```python
from build123d import *

# Parameters (mm, degrees)
F1_DEPTH     = 2.54
F3_DEPTH     = 2.54
F4_R         = 2.9314454593
F5_R         = 2.8319389427
F6_DEPTH     = 8.89
F8_DEPTH     = 25.4
F9_T1_DEPTH  = 38.1
F9_T3_DEPTH  = 38.1
F9_T5_DEPTH  = 21.5282681004
F9_T7_DEPTH  = 32.0580135728
F9_T9_DEPTH  = 55.7565362009
F9_T11_DEPTH = 34.6970452561
F9_T13_DEPTH = 34.6970452561
F9_T16_ANGLE = 223.4050528115
F9_T21_DEPTH = 49.0985226281
F9_T25_DEPTH = 32.5267907285
F9_T32_DEPTH = 32.0580135728
F9_T37_DEPTH = 49.0985226281
F9_T44_DEPTH = 49.0985226281
F9_T48_DEPTH = 32.0580135728
F9_T56_DEPTH = 32.5267907285
F9_T60_DEPTH = 49.0985226281
F10_R        = 1.4567648878
F10_R_2      = 1.5876943873
F11_DEPTH    = 0.508
F12_R        = 0.6244535606
F12_R_2      = 0.645662674
F13_DEPTH    = 0.254


# Not quite as in the source:
# - a fillet or chamfer that OpenCascade refuses, or shapes differently, is made with other operations: its cross-section is extruded or revolved along the edge and cut away or added


with BuildPart() as f1:
    # F0 (on Front) → F1 (new body)
    with BuildSketch(Plane.XZ):
        Polygon((27.5468391635, 41.7749450469), (-86.7531608365, 41.7749450469), (-86.7531608365, 8.0154541022), (-74.0531608365, 8.0154541022), (-74.0531608365, 29.0749450469), (-35.9531608365, 29.0749450469), (-35.9531608365, 8.0154541022), (-23.2531608365, 8.0154541022), (-23.2531608365, 29.0749450469), (14.8468391635, 29.0749450469), (14.8468391635, 8.0154541022), (27.5468391635, 8.0154541022), align=None)
    extrude(amount=F1_DEPTH)

    # F2 (on face) → F3 (join)
    with BuildSketch(Plane.XY.offset(41.7749450469)):
        with BuildLine():
            Line((27.5468391635, -2.54), (13.0688391635, -2.54))
            ThreePointArc((13.0688391635, -2.54), (20.3078391635, -9.779), (27.5468391635, -2.54))
        make_face()
        with BuildLine():
            Line((-72.2751608365, -2.54), (-86.7531608365, -2.54))
            ThreePointArc((-86.7531608365, -2.54), (-79.5141608365, -9.779), (-72.2751608365, -2.54))
        make_face()
    extrude(amount=-F3_DEPTH)

    # F4 (on face) + F5 (on face) → F6 (join)
    with BuildSketch(Plane(origin=(0, 0, 39.2349450469), x_dir=(1, 0, 0), z_dir=(0, 0, -1))):
        with Locations((-79.5141608365, 6.3278437592)):
            Circle(F4_R)
    with BuildSketch(Plane(origin=(0, 0, 39.2349450469), x_dir=(1, 0, 0), z_dir=(0, 0, -1))):
        with Locations((20.3078391635, 6.6598863341)):
            Circle(F5_R)
    extrude(amount=F6_DEPTH)

    # F7 (on face) → F8 (cut)
    with BuildSketch(Plane.XZ.offset(2.54)):
        with BuildLine():
            Line((-23.2531608365, 8.0154541022), (-23.2531608365, 18.5451995745))
            ThreePointArc((-23.2531608365, 18.5451995745), (-29.6031608365, 21.0747577819), (-35.9531608365, 18.5451995745))
            Line((-35.9531608365, 18.5451995745), (-35.9531608365, 8.0154541022))
            Line((-35.9531608365, 8.0154541022), (-23.2531608365, 8.0154541022))
        make_face()
    extrude(amount=-F8_DEPTH, mode=Mode.SUBTRACT)

    # F9: fillet of radius 5.08 on 11 edges, made by hand

    # F9_s2 → F9_t1 (cut)
    with BuildSketch(Plane.YZ.offset(-23.2531608365)):
        with BuildLine():
            ThreePointArc((0, 33.4743540981), (-0.6805909488, 30.9343540981), (-2.54, 29.0749450469))
            Line((-2.54, 29.0749450469), (0, 29.0749450469))
            Line((0, 29.0749450469), (0, 33.4743540981))
        make_face()
    extrude(amount=F9_T1_DEPTH, mode=Mode.SUBTRACT)

    # F9_s4 → F9_t3 (cut)
    with BuildSketch(Plane.YZ.offset(-74.0531608365)):
        with BuildLine():
            ThreePointArc((0, 33.4743540981), (-0.6805909488, 30.9343540981), (-2.54, 29.0749450469))
            Line((-2.54, 29.0749450469), (0, 29.0749450469))
            Line((0, 29.0749450469), (0, 33.4743540981))
        make_face()
    extrude(amount=F9_T3_DEPTH, mode=Mode.SUBTRACT)

    # F9_s6 → F9_t5 (cut)
    with BuildSketch(Plane.XY.offset(7.5466769465)):
        with BuildLine():
            ThreePointArc((-31.5537517853, 0), (-34.0937517853, -0.6805909488), (-35.9531608365, -2.54))
            Line((-35.9531608365, -2.54), (-35.9531608365, 0))
            Line((-35.9531608365, 0), (-31.5537517853, 0))
        make_face()
        with BuildLine():
            ThreePointArc((-27.6525698878, 0), (-25.1125698878, -0.6805909488), (-23.2531608365, -2.54))
            Line((-23.2531608365, -2.54), (-23.2531608365, 0))
            Line((-23.2531608365, 0), (-27.6525698878, 0))
        make_face()
    extrude(amount=F9_T5_DEPTH, mode=Mode.SUBTRACT)

    # F9_s8 → F9_t7 (cut)
    with BuildSketch(Plane.XY.offset(-2.9830685259)):
        with BuildLine():
            ThreePointArc((19.2462482147, 0), (16.7062482147, -0.6805909488), (14.8468391635, -2.54))
            Line((14.8468391635, -2.54), (14.8468391635, 0))
            Line((14.8468391635, 0), (19.2462482147, 0))
        make_face()
        with BuildLine():
            ThreePointArc((-78.4525698878, 0), (-75.9125698878, -0.6805909488), (-74.0531608365, -2.54))
            Line((-74.0531608365, -2.54), (-74.0531608365, 0))
            Line((-74.0531608365, 0), (-78.4525698878, 0))
        make_face()
    extrude(amount=F9_T7_DEPTH, mode=Mode.SUBTRACT)

    # F9_s10 → F9_t9 (cut)
    with BuildSketch(Plane.XY.offset(-2.9830685259)):
        with BuildLine():
            ThreePointArc((27.5468391635, -2.54), (25.6874301122, -0.6805909488), (23.1474301122, 0))
            Line((23.1474301122, 0), (27.5468391635, 0))
            Line((27.5468391635, 0), (27.5468391635, -2.54))
        make_face()
        with BuildLine():
            ThreePointArc((-86.7531608365, -2.54), (-84.8937517853, -0.6805909488), (-82.3537517853, 0))
            Line((-82.3537517853, 0), (-86.7531608365, 0))
            Line((-86.7531608365, 0), (-86.7531608365, -2.54))
        make_face()
    extrude(amount=F9_T9_DEPTH, mode=Mode.SUBTRACT)

    # F9_s12 → F9_t11 (cut)
    with BuildSketch(Plane.YZ.offset(-97.7516834646)):
        with BuildLine():
            ThreePointArc((0, 12.4148631534), (-0.6805909488, 9.8748631534), (-2.54, 8.0154541022))
            Line((-2.54, 8.0154541022), (0, 8.0154541022))
            Line((0, 8.0154541022), (0, 12.4148631534))
        make_face()
    extrude(amount=F9_T11_DEPTH, mode=Mode.SUBTRACT)

    # F9_s14 → F9_t13 (cut)
    with BuildSketch(Plane.YZ.offset(3.8483165354)):
        with BuildLine():
            ThreePointArc((0, 12.4148631534), (-0.6805909488, 9.8748631534), (-2.54, 8.0154541022))
            Line((-2.54, 8.0154541022), (0, 8.0154541022))
            Line((0, 8.0154541022), (0, 12.4148631534))
        make_face()
    extrude(amount=F9_T13_DEPTH, mode=Mode.SUBTRACT)

    # F9_s15 → F9_t16 (revolve, cut)
    with BuildSketch(Plane(origin=(0.0198149882, 0, 0.0497864763), x_dir=(0, 1, 0), z_dir=(-0.3697877262, 0, -0.929116267))):
        with BuildLine():
            ThreePointArc((0, -18.2485055237), (-0.6805909488, -20.7885055237), (-2.54, -22.6479145749))
            Line((-2.54, -22.6479145749), (0, -22.6479145749))
            Line((0, -22.6479145749), (0, -18.2485055237))
        make_face()
    revolve(axis=Axis((-29.6031608365, 0, 11.8397133801), (0, -1, 0)), revolution_arc=F9_T16_ANGLE, mode=Mode.SUBTRACT)


with BuildPart() as f9_tool19:
    # F9_s20 → F9_t21 (new body)
    with BuildSketch(Plane.YZ.offset(-34.2516834646)):
        with BuildLine():
            ThreePointArc((0, 33.4743540981), (-0.6805909488, 30.9343540981), (-2.54, 29.0749450469))
            Line((-2.54, 29.0749450469), (0, 29.0749450469))
            Line((0, 29.0749450469), (0, 33.4743540981))
        make_face()
    extrude(amount=F9_T21_DEPTH)

    split(bisect_by=Plane.YZ.offset(-23.2531608365), keep=Keep.BOTTOM)


with BuildPart() as f9_tool23:
    # F9_s24 → F9_t25 (new body)
    with BuildSketch(Plane.XY.offset(7.5466769465)):
        with BuildLine():
            ThreePointArc((-27.6525698878, 0), (-25.1125698878, -0.6805909488), (-23.2531608365, -2.54))
            Line((-23.2531608365, -2.54), (-23.2531608365, 0))
            Line((-23.2531608365, 0), (-27.6525698878, 0))
        make_face()
    extrude(amount=F9_T25_DEPTH)

    split(bisect_by=Plane.XY.offset(29.0749450469), keep=Keep.TOP)


with BuildPart() as f9_tool19_1:
    add(f9_tool19.part)

    # F9_t27: intersect F9_tool23
    add(f9_tool23.part, mode=Mode.INTERSECT)


with BuildPart() as f1_1:
    add(f1.part)

    # F9_t17: cut F9_tool19
    add(f9_tool19_1.part, mode=Mode.SUBTRACT)


with BuildPart() as f9_tool30:
    # F9_s31 → F9_t32 (new body)
    with BuildSketch(Plane.XY.offset(40.073467675)):
        with BuildLine():
            ThreePointArc((19.2462482147, 0), (16.7062482147, -0.6805909488), (14.8468391635, -2.54))
            Line((14.8468391635, -2.54), (14.8468391635, 0))
            Line((14.8468391635, 0), (19.2462482147, 0))
        make_face()
    extrude(amount=-F9_T32_DEPTH)

    split(bisect_by=Plane.XY.offset(39.2349450469), keep=Keep.BOTTOM)

    split(bisect_by=Plane.XY.offset(29.0749450469), keep=Keep.TOP)


with BuildPart() as f9_tool35:
    # F9_s36 → F9_t37 (new body)
    with BuildSketch(Plane.YZ.offset(-23.2531608365)):
        with BuildLine():
            ThreePointArc((0, 33.4743540981), (-0.6805909488, 30.9343540981), (-2.54, 29.0749450469))
            Line((-2.54, 29.0749450469), (0, 29.0749450469))
            Line((0, 29.0749450469), (0, 33.4743540981))
        make_face()
    extrude(amount=F9_T37_DEPTH)

    split(bisect_by=Plane.YZ.offset(14.8468391635), keep=Keep.TOP)


with BuildPart() as f9_tool30_1:
    add(f9_tool30.part)

    # F9_t39: intersect F9_tool35
    add(f9_tool35.part, mode=Mode.INTERSECT)


with BuildPart() as f1_2:
    add(f1_1.part)

    # F9_t28: cut F9_tool30
    add(f9_tool30_1.part, mode=Mode.SUBTRACT)


with BuildPart() as f9_tool42:
    # F9_s43 → F9_t44 (new body)
    with BuildSketch(Plane.YZ.offset(-85.0516834646)):
        with BuildLine():
            ThreePointArc((0, 33.4743540981), (-0.6805909488, 30.9343540981), (-2.54, 29.0749450469))
            Line((-2.54, 29.0749450469), (0, 29.0749450469))
            Line((0, 29.0749450469), (0, 33.4743540981))
        make_face()
    extrude(amount=F9_T44_DEPTH)

    split(bisect_by=Plane.YZ.offset(-74.0531608365), keep=Keep.BOTTOM)


with BuildPart() as f9_tool46:
    # F9_s47 → F9_t48 (new body)
    with BuildSketch(Plane.XY.offset(8.0154541022)):
        with BuildLine():
            ThreePointArc((-78.4525698878, 0), (-75.9125698878, -0.6805909488), (-74.0531608365, -2.54))
            Line((-74.0531608365, -2.54), (-74.0531608365, 0))
            Line((-74.0531608365, 0), (-78.4525698878, 0))
        make_face()
    extrude(amount=F9_T48_DEPTH)

    split(bisect_by=Plane.XY.offset(29.0749450469), keep=Keep.TOP)

    split(bisect_by=Plane.XY.offset(39.2349450469), keep=Keep.BOTTOM)


with BuildPart() as f9_tool42_1:
    add(f9_tool42.part)

    # F9_t51: intersect F9_tool46
    add(f9_tool46.part, mode=Mode.INTERSECT)


with BuildPart() as f1_3:
    add(f1_2.part)

    # F9_t40: cut F9_tool42
    add(f9_tool42_1.part, mode=Mode.SUBTRACT)


with BuildPart() as f9_tool54:
    # F9_s55 → F9_t56 (new body)
    with BuildSketch(Plane.XY.offset(40.073467675)):
        with BuildLine():
            ThreePointArc((-31.5537517853, 0), (-34.0937517853, -0.6805909488), (-35.9531608365, -2.54))
            Line((-35.9531608365, -2.54), (-35.9531608365, 0))
            Line((-35.9531608365, 0), (-31.5537517853, 0))
        make_face()
    extrude(amount=-F9_T56_DEPTH)

    split(bisect_by=Plane.XY.offset(29.0749450469), keep=Keep.TOP)


with BuildPart() as f9_tool58:
    # F9_s59 → F9_t60 (new body)
    with BuildSketch(Plane.YZ.offset(-74.0531608365)):
        with BuildLine():
            ThreePointArc((0, 33.4743540981), (-0.6805909488, 30.9343540981), (-2.54, 29.0749450469))
            Line((-2.54, 29.0749450469), (0, 29.0749450469))
            Line((0, 29.0749450469), (0, 33.4743540981))
        make_face()
    extrude(amount=F9_T60_DEPTH)

    split(bisect_by=Plane.YZ.offset(-35.9531608365), keep=Keep.TOP)


with BuildPart() as f9_tool54_1:
    add(f9_tool54.part)

    # F9_t62: intersect F9_tool58
    add(f9_tool58.part, mode=Mode.INTERSECT)


with BuildPart() as f1_4:
    add(f1_3.part)

    # F9_t52: cut F9_tool54
    add(f9_tool54_1.part, mode=Mode.SUBTRACT)

    # F10 (on Front) → F11 (cut)
    with BuildSketch(Plane.XZ):
        with Locations((21.32573165, 15.5286919326)):
            Circle(F10_R)
        with Locations((-80.219194293, 15.5286919326)):
            Circle(F10_R_2)
    extrude(amount=F11_DEPTH, mode=Mode.SUBTRACT)

    # F12 (on face) → F13 (join)
    with BuildSketch(Plane(origin=(0, -0.508, 0), x_dir=(-1, 0, 0), z_dir=(0, 1, 0))):
        with Locations((-21.32573165, 15.5286919326)):
            Circle(F12_R)
        with Locations((80.0827890635, 15.5286919326)):
            Circle(F12_R_2)
    extrude(amount=F13_DEPTH)


solid = f1_4.part
```
Model file for the job. Use its own axes, mm. A direction names the side the tool comes from. Give positions to 0.01 mm unless a question says otherwise; leave off trailing zeros. Loops run counter-clockwise (first coordinate to the right, second up) from the corner with the lowest first, then second, coordinate; pieces in that order, holes last. Notation, with made-up numbers: (-35.5, -6.5) - (-26.5, -6.5) arc R35 ccw to (-26.5, 25.5) - close; hole circle Ø10 at (67, 15.5). An arc over 180 degrees is marked (long way). One line per item, written item: value. Start each with the question number.
1. Probe L1, parallel to X at y = -3, z = 40; L2, parallel to Y at x = -80.5, z = 28.5; L3, parallel to Z at x = 21.5, y = -9.5. List the from-to ranges inside material, lowest first. Write a range as from..to.
2. Slice it at B-B (x = -62.5). List the corners of the cut face in (y, z).
3. Slice it at A-A (z = 22). Give the number of separate pieces and of enclosed holes in the cut face, plus the area to 3 significant figures.
4. Pull direction X, two halves, no side cores. Call faces 1 (the flat face through (22, -4, 39.235)), 2 (the flat face through (20, -7, 30.345)), 3 (the cylindrical face through (-84.93, -0.7, 24.66)): pulls with the +X half, pulls with the -X half, needs draft (parallel to the pull), parting line crosses it, or undercut.
5. Pin check, flat tips, straight feed: pin 1 (1.8 mm diameter, centred on x = -79.5, y = -7, fed in from -Z); pin 2 (2 mm diameter, centred on y = -3.5, z = 28, fed in from +X); pin 3 (1 mm diameter, centred on y = -5, z = 25.5, fed in from +X); pin 4 (0.9 mm diameter, centred on x = 21, z = 15.5, fed in from +Y). Stop position of each tip, or through.
6. Which spindle directions (+Z, -Z, +X, -X, +Y, -Y) get a long thin tool onto all of the face, cutting with end or side? Do faces 4 (the cylindrical face through (-34.06, -0.66, 25.91)), 5 (the flat face through (-80, -6, 30.345)), 6 (the cylindrical face through (-81.805, -0.25, 15.598)). Say none if no direction does.
Solution:
1. L1: x = -86.74..-72.29, 13.08..27.53
1. L2: y = -2.54..0
1. L3: z = 39.23..41.77
2. outline: (-2.54, 29.07) arc R5.08 ccw to (0, 33.47) - (0, 41.77) - (-2.54, 41.77) - close
3. separate pieces: 3
3. enclosed holes: 0
3. area: 68.4 mm^2
4. face 1: undercut
4. face 2: needs draft
4. face 3: pulls with the -X half
5. pin 1: stops at z = 30.34
5. pin 2: stops at x = 27.55
5. pin 3: passes through
5. pin 4: stops at y = -0.25
6. face 4: -Z, +Y
6. face 5: -Z, +X, -X, -Y
6. face 6: +Y
